Verification items for the finished model (mm, model axes). A direction names the side the tool comes from. Round coordinates to 2 decimals unless told otherwise and drop trailing zeros. Order: outer loops, then holes, each group sorted by start corner. A loop starts at its lowest first (then second) coordinate and runs counter-clockwise, first axis right, second up.
```python
from build123d import *

# Parameters (mm, degrees)
RESSALTO_EXTRUS_O1_DEPTH = 1000
ESBO_O2_R                = 20
RESSALTO_EXTRUS_O2_DEPTH = 30


with BuildPart() as part:
    # Esboço1 → Ressalto-extrusão1 (new body, symmetric)
    with BuildSketch(Plane(origin=(0, 0, 0), x_dir=(0, 0, -1), z_dir=(1, 0, 0))):
        Polygon((-40, 80), (40, 80), (40, 30), (100, 30), (100, 0), (-100, 0), (-100, 30), (-40, 30), align=None)
    extrude(amount=RESSALTO_EXTRUS_O1_DEPTH, both=True)

    # Esboço2 → Ressalto-extrusão2 (add)
    with BuildSketch(Plane(origin=(0, 0, 0), x_dir=(-1, 0, 0), z_dir=(0, -1, 0))):
        Circle(ESBO_O2_R)
    extrude(amount=RESSALTO_EXTRUS_O2_DEPTH)


solid = part.part
```
1) Go/stop test with flat-tipped pins: pin 1 Ø1.5 at (x, z) = (472, 0) entering from -Y; pin 2 Ø4 at (x, y) = (135, 40.5) entering from +Z; pin 3 Ø8 at (x, z) = (743, 42.5) entering from +Y. Record where each tip stops, or that it passes through.
2) Tool access check on faces 1 (the flat face through (14, 30, -70)), 2 (the flat face through (14, 30, 70)), 3 (the cylindrical face through (4.336, -14.79, 19.524)). Record the directions out of +Z, -Z, +X, -X, +Y, -Y that give a thin tool (end or side, any length) a straight path to the whole face; none if there is none.
3) Scan lines: probe 1 along Y at (x, z) = (-705.5, 73); probe 2 along Z at (x, y) = (-679, 53.5); probe 3 along Y at (x, z) = (479, -15). Record each from-to range of solid material in increasing order.
4) Sectioned sample at C-C on y = 54. Record the cut outline in (x, z), then the cut area to 3 significant figures.
5) Sectioned sample at D-D on x = -422. Record the cut outline in (y, z).
6) Sectioned sample at B-B on z = 0. Record the cut outline in (x, y), then the cut area to 3 significant figures.
7) Sectioned sample at A-A on x = 0. Record the cut outline in (y, z).
Returned:
1. pin 1: stops at y = 0
1. pin 2: stops at z = 40
1. pin 3: stops at y = 80
2. face 1: -Z, +X, -X, +Y
2. face 2: +Z, +X, -X, +Y
2. face 3: -Y
3. probe 1: y = 0 to 30
3. probe 2: z = -40 to 40
3. probe 3: y = 0 to 80
4. outline: (-1000, -40) - (1000, -40) - (1000, 40) - (-1000, 40) - close
4. area: 160,000 mm2
5. outline: (0, -100) - (30, -100) - (30, -40) - (80, -40) - (80, 40) - (30, 40) - (30, 100) - (0, 100) - close
6. outline: (-1000, 0) - (-20, 0) - (-20, -30) - (20, -30) - (20, 0) - (1000, 0) - (1000, 80) - (-1000, 80) - close
6. area: 161,000 mm2
7. outline: (-30, -20) - (0, -20) - (0, -100) - (30, -100) - (30, -40) - (80, -40) - (80, 40) - (30, 40) - (30, 100) - (0, 100) - (0, 20) - (-30, 20) - close
